```python
from build123d import *

# Parameters (mm, degrees)
SKETCH_1_R               = 9.975
EXTRUDE_1_DEPTH          = 4
SKETCH_2_R               = 1.5
CUT_EXTRUDE_1_DEPTH      = 15.662920923
PATTERN_CIRCULAR_1_COUNT = 4
SKETCH_3_R               = 3
CUT_EXTRUDE_2_DEPTH      = 15.662920923


with BuildPart() as part:
    # 草图1 → 凸台-拉伸1 (new body)
    with BuildSketch(Plane.XY):
        Circle(SKETCH_1_R)
    extrude(amount=EXTRUDE_1_DEPTH)

    # 草图2 → 切除-拉伸1 (cut, through all)
    with BuildSketch(Plane.XY.offset(4)):
        with Locations((-7, 0)):
            Circle(SKETCH_2_R)
    cut_extrude_1 = extrude(amount=-CUT_EXTRUDE_1_DEPTH, mode=Mode.SUBTRACT)

    # 阵列(圆周)1: 切除-拉伸1 ×4 about axis
    pattern_circular_1_axis = Axis((0, 0, 0), (0, 0, 1))
    for i in range(1, PATTERN_CIRCULAR_1_COUNT):
        add(cut_extrude_1.rotate(pattern_circular_1_axis, i * 360 / PATTERN_CIRCULAR_1_COUNT), mode=Mode.SUBTRACT)

    # 草图3 → 切除-拉伸2 (cut, through all)
    with BuildSketch(Plane.XY.offset(4)):
        Circle(SKETCH_3_R)
    extrude(amount=-CUT_EXTRUDE_2_DEPTH, mode=Mode.SUBTRACT)


solid = part.part
```
Geometry: final body of the model. Coordinates: model frame, mm. Coordinates: 2 decimals unless noted, no trailing zeros. Write each loop counter-clockwise with the first axis right and the second up, starting at its lowest first coordinate (ties: lowest second). Pieces come first, ordered by that corner, then holes. Notation, with made-up numbers: M 89.25,59 L 135.25,59 A13 cw 135.25,64 Z; hole C 40.25,55.25 d10. An arc over 180 degrees is marked long. Use CSV: the item, a comma, the result in double quotes. Start each with the question number.
1. Cut plane B-B on y = 0.75. Return the cut outline in (x, z), plus the area to 3 significant figures.
2. Mould query, pull axis X, two halves, no side actions, for faces 1 (the face through (0.07, 8.5, 2.03)), 2 (the face through (9.514, 2.996, 1.972)), 3 (the face through (-2.4, -2.1, 4)). Classes: pulls with the +X half, pulls with the -X half, needs draft (parallel to the pull), parting line crosses it, or undercut.
3. First-contact query: P1, Ø2, axis at y = -1.5, z = 1, coming from the +X side; P2, Ø5, axis at x = -7, y = 0, coming from the -Z side; P3, Ø2, axis at y = -4, z = 2.5, coming from the -X side; P4, Ø1.5, axis at x = 5, z = 1, coming from the +Y side. Flat tips, straight axial feed; report the tip coordinate or a pass-through.
4. Ray query, probe 1 along X at (y, z) = (-0.25, 3.75); probe 2 along X at (y, z) = (1.25, 2.45); probe 3 along Y at (x, z) = (1, 3.7). Return the intervals inside material, ascending.
5. Cut plane A-A on x = 0. Return the cut outline in (y, z) (3 decimals), plus the area to 3 significant figures.
6. Cut plane D-D on y = -7. Return the cut outline in (x, z).
7. Cut plane C-C on z = 1.45. Return the cut outline in (x, y) (3 decimals), plus the area to 3 significant figures.
Entries:
1,outline,"M -9.95,0 L -8.3,0 L -8.3,4 L -9.95,4 Z; M -5.7,0 L -2.9,0 L -2.9,4 L -5.7,4 Z; M 2.9,0 L 5.7,0 L 5.7,4 L 2.9,4 Z; M 8.3,0 L 9.95,0 L 9.95,4 L 8.3,4 Z"
1,area,"35.6 mm²"
2,face 1,"undercut"
2,face 2,"parting line crosses it"
2,face 3,"needs draft"
3,P1,"x = 9.96"
3,P2,"z = 0"
3,P3,"x = -9.51"
3,P4,"y = 9.02"
4,probe 1,"-9.97 to -8.48, -5.52 to -2.99, 2.99 to 5.52, 8.48 to 9.97"
4,probe 2,"-9.9 to -7.83, -6.17 to -2.73, 2.73 to 6.17, 7.83 to 9.9"
4,probe 3,"-9.92 to -8.12, -5.88 to -2.83, 2.83 to 5.88, 8.12 to 9.92"
5,outline,"M -9.975,0 L -8.5,0 L -8.5,4 L -9.975,4 Z; M -5.5,0 L -3,0 L -3,4 L -5.5,4 Z; M 3,0 L 5.5,0 L 5.5,4 L 3,4 Z; M 8.5,0 L 9.975,0 L 9.975,4 L 8.5,4 Z"
5,area,"31.8 mm²"
6,outline,"M -7.11,0 L -1.5,0 L -1.5,4 L -7.11,4 Z; M 1.5,0 L 7.11,0 L 7.11,4 L 1.5,4 Z"
7,outline,"C 0,0 d19.95; hole C -7,0 d3; hole C 0,0 d6; hole C 0,-7 d3; hole C 0,7 d3; hole C 7,0 d3"
7,area,"256 mm²"
